The listing builds one solid part. Answer for the finished solid, in the listing's coordinates (mm). A direction names the side the tool comes from. Coordinates: 2 decimals unless noted, no trailing zeros. Write each loop counter-clockwise with the first axis right and the second up, starting at its lowest first coordinate (ties: lowest second). Pieces come first, ordered by that corner, then holes. Notation, with made-up numbers: M 66,-39 L 107,-39 A31 cw 107,-12 Z; hole C 21,15 d2. An arc over 180 degrees is marked long. Answer as a JSON object with one key per item and string values. Group by question number.
from build123d import *

# Parameters (mm, degrees)
CYLINDER024_R             = 41.25
CYLINDER024_DEPTH         = 1.5
BOX_W                     = 16.9
BOX_H                     = 4
BOX_DEPTH                 = 1.5
BOX001_W                  = 16.9
BOX001_H                  = 4
BOX001_DEPTH              = 1.5
FUSION007_PLACEMENT_ANGLE = 22.5
CYLINDER003_R             = 4.2
CYLINDER003_DEPTH         = 17
ARRAY_COUNT               = 8
CYLINDER002_R             = 38.6
CYLINDER002_DEPTH         = 0.22
CYLINDER001_R             = 41.25
CYLINDER001_DEPTH         = 1.2
CYLINDER_R                = 57.15
CYLINDER_DEPTH            = 17


with BuildPart() as cylinder024:
    # Cylinder024 → Cylinder024 (new body)
    with BuildSketch(Plane.XY):
        Circle(CYLINDER024_R)
    extrude(amount=CYLINDER024_DEPTH)


with BuildPart() as cube:
    # Box → Box (new body)
    with BuildSketch(Plane(origin=(40.75, -2, 0), x_dir=(1, 0, 0), z_dir=(0, 0, 1))):
        with Locations((8.45, 2)):
            Rectangle(BOX_W, BOX_H)
    extrude(amount=BOX_DEPTH)


with BuildPart() as obj1:
    # Box001 → Box001 (new body)
    with BuildSketch(Plane(origin=(-57.65, -2, 0), x_dir=(1, 0, 0), z_dir=(0, 0, 1))):
        with Locations((8.45, 2)):
            Rectangle(BOX001_W, BOX001_H)
    extrude(amount=BOX001_DEPTH)

    # Fusion007: union Cube
    add(cube.part)


with BuildPart() as obj1_1:
    # Fusion007 placement: moved
    add(obj1.part.rotate(Axis((0, 0, 0), (0, 0, 1)), FUSION007_PLACEMENT_ANGLE))

    # Cut019: cut Cylinder024
    add(cylinder024.part, mode=Mode.SUBTRACT)


with BuildPart() as boltholearray:
    # Cylinder003 → Cylinder003 (new body)
    with BuildSketch(Plane(origin=(46.1, 0, 0), x_dir=(1, 0, 0), z_dir=(0, 0, 1))):
        Circle(CYLINDER003_R)
    extrude(amount=CYLINDER003_DEPTH)

    # Array: BoltHoleArray ×8 about axis
    array_axis = Axis((0, 0, 0), (0, 0, 1))


with BuildPart() as boltholearray_1:
    add(boltholearray.part)
    for i in range(1, ARRAY_COUNT):
        add(boltholearray.part.rotate(array_axis, i * 360 / ARRAY_COUNT))


with BuildPart() as cylinder:
    # Cylinder002 → Cylinder002 (new body)
    with BuildSketch(Plane.XY):
        Circle(CYLINDER002_R)
    extrude(amount=CYLINDER002_DEPTH)


with BuildPart() as knifeedge:
    # Cone → Cone (revolve)
    with BuildSketch(Plane.XZ):
        Polygon((0, 0), (38.6, 0), (41.25, 0.22), (0, 0.22), align=None)
    revolve(axis=Axis((0, 0, 0), (0, 0, 1)))

    # Cut001: cut Cylinder
    add(cylinder.part, mode=Mode.SUBTRACT)


with BuildPart() as knifeedge_1:
    # Cut001 placement: moved
    add(knifeedge.part.moved(Location((0, 0, 0.98))))


with BuildPart() as sealrecess:
    # Cylinder001 → Cylinder001 (new body)
    with BuildSketch(Plane.XY):
        Circle(CYLINDER001_R)
    extrude(amount=CYLINDER001_DEPTH)


with BuildPart() as obj2:
    # Cylinder → Cylinder (new body)
    with BuildSketch(Plane.XY):
        Circle(CYLINDER_R)
    extrude(amount=CYLINDER_DEPTH)

    # Cut: cut SealRecess
    add(sealrecess.part, mode=Mode.SUBTRACT)

    # Fusion: union KnifeEdge
    add(knifeedge_1.part)

    # Cut002: cut BoltHoleArray
    add(boltholearray_1.part, mode=Mode.SUBTRACT)

    # Cut020: cut obj1
    add(obj1_1.part, mode=Mode.SUBTRACT)


solid = obj2.part
Item 1: A cutting plane is placed at C-C, the plane x = 46.1. Write down the section's boundary in (y, z), and give its area (3 significant figures).
Item 2: A cutting plane is placed at A-A, the plane y = 0. Write down the section's boundary in (x, z), and give its area (3 significant figures).
Item 3: Consider L1, parallel to Y at x = 35.5, z = 3; L2, parallel to Y at x = -29.5, z = 9.75; L3, parallel to Z at x = 4, y = 1.5. Determine where each line is inside the solid, lowest interval first. Write a range as from..to.
Item 4: A tool of negligible diameter and unlimited length cuts with its end or side. For faces 1 (the face through (-14.97, 38.438, 0.592)), 2 (the face through (-29.76, 29.5, 8.38)), from which of +Z, -Z, +X, -X, +Y, -Y can it reach the whole face along a straight path? Write none if from no direction.
Item 5: Flat-ended cylindrical pins translate along their axes: pin 1 Ø9.5 at (x, y) = (32.6, -32.6) entering from -Z; pin 2 Ø3 at (y, z) = (-26.5, 11.5) entering from -X; pin 3 Ø4 at (x, z) = (-16.5, 8) entering from +Y; pin 4 Ø2 at (x, z) = (10.5, 15) entering from -Y. Find the tip coordinate at first contact, or state that the pin passes through.
Item 6: A cutting plane is placed at D-D, the plane z = 14.5. State how many separate pieces and enclosed holes the cut face has, and give its area (3 significant figures).
Answer:
{
 "1": {"outline": "M -33.78,0 L -4.2,0 L -4.2,17 L -33.78,17 Z; M 4.2,0 L 16.93,0 L 16.93,1.5 L 21.26,1.5 L 21.26,0 L 33.78,0 L 33.78,17 L 4.2,17 Z", "area": "999 mm2"},
 "2": {"outline": "M -57.15,0 L -50.3,0 L -50.3,17 L -57.15,17 Z; M -41.9,0 L -41.25,0 L -41.25,1.2 L -38.6,0.98 L -38.6,1.2 L 38.6,1.2 L 38.6,0.98 L 41.25,1.2 L 41.25,0 L 41.9,0 L 41.9,17 L -41.9,17 Z; M 50.3,0 L 57.15,0 L 57.15,17 L 50.3,17 Z", "area": "1,560 mm2"},
 "3": {"L1": "-44.79..-35.63, -29.56..29.56, 35.63..44.79", "L2": "-48.95..-35.43, -29.76..29.76, 35.43..48.95", "L3": "1.2..17"},
 "4": {"face 1": "-Z", "face 2": "+Z, -Z"},
 "5": {"pin 1": "z = 0", "pin 2": "x = -51.39", "pin 3": "y = 55.28", "pin 4": "y = -56.35"},
 "6": {"separate pieces": "1", "enclosed holes": "8", "area": "9,820 mm2"}
}
